Part print with two shaded views. Sizes in mm from the minimum x, y, z corner. A direction names the side the tool comes from. Give positions to 0.01 mm unless a question says otherwise; leave off trailing zeros. Order: outer loops, then holes, each group sorted by start corner. A loop starts at its lowest first (then second) coordinate and runs counter-clockwise, first axis right, second up. Notation, with made-up numbers: (54, -34.5) -> (76, -34.5) arc R31 cw to (76, 0.5) -> close; hole circle Ø6 at (-25, -40). An arc over 180 degrees is marked (long way). Answer as CSV lines item,"result".
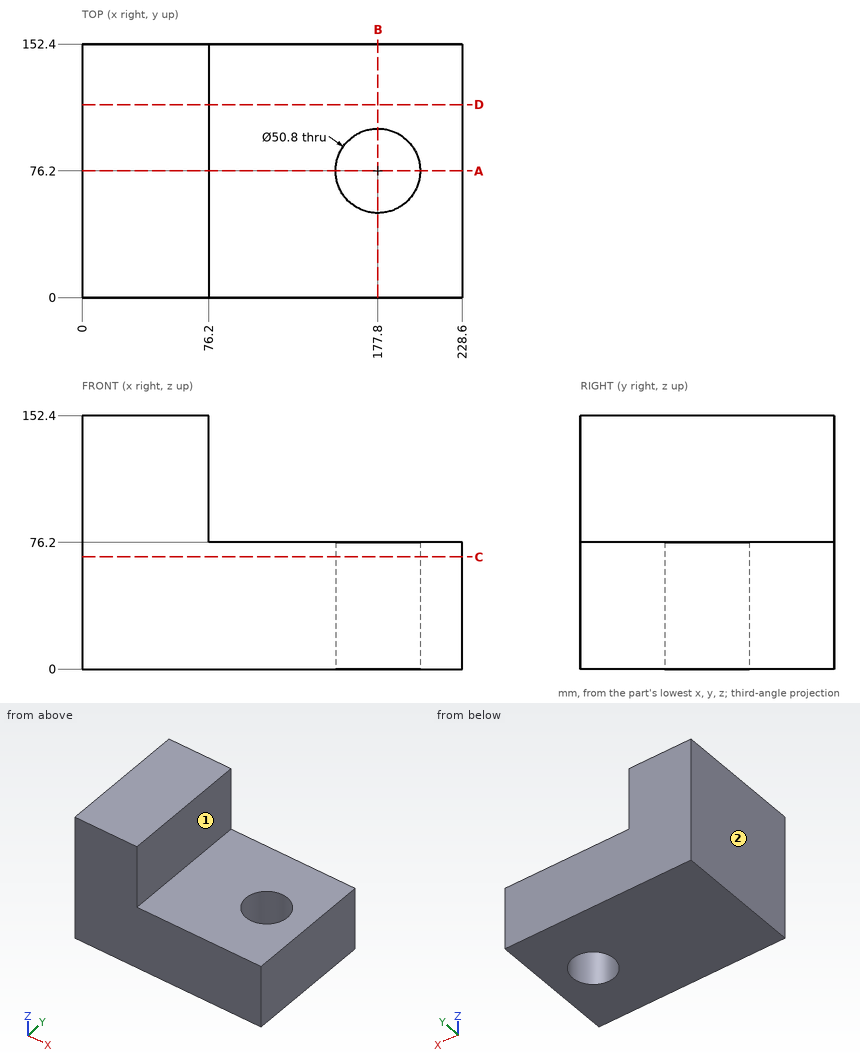
1) Which spindle directions (+Z, -Z, +X, -X, +Y, -Y) get a long thin tool onto all of the face, cutting with end or side? Do the marked faces 1 and 2. Say none if no direction does.
Data:
face 1,"+Z, +X, +Y, -Y"
face 2,"+Z, -Z, -X, +Y, -Y"
2) Wall check: line 1 along Y through (x, z) = (177.8, 44.5); line 2 along X through (y, z) = (40, 91.5); line 3 along X through (y, z) = (76, 48). Give the ranges that are in metal, low to high. Write a range as [from, to].
Data:
line 1,"y = [0, 50.8], [101.6, 152.4]"
line 2,"x = [0, 76.2]"
line 3,"x = [0, 152.4], [203.2, 228.6]"
3) Band-saw the part on A-A, the plane y = 76.2. Write the cut outline in (x, z), then the cut area to 3 significant figures.
Data:
outline,"(0, 0) -> (152.4, 0) -> (152.4, 76.2) -> (76.2, 76.2) -> (76.2, 152.4) -> (0, 152.4) -> close; (203.2, 0) -> (228.6, 0) -> (228.6, 76.2) -> (203.2, 76.2) -> close"
area,"19,400 mm2"
4) Band-saw the part on C-C, the plane z = 67.5. Write the cut outline in (x, y).
Data:
outline,"(0, 0) -> (228.6, 0) -> (228.6, 152.4) -> (0, 152.4) -> close; hole circle Ø50.8 at (177.8, 76.2)"
5) Band-saw the part on B-B, the plane x = 177.8. Write the cut outline in (y, z), then the cut area to 3 significant figures.
Data:
outline,"(0, 0) -> (50.8, 0) -> (50.8, 76.2) -> (0, 76.2) -> close; (101.6, 0) -> (152.4, 0) -> (152.4, 76.2) -> (101.6, 76.2) -> close"
area,"7,740 mm2"
6) Band-saw the part on D-D, the plane y = 116. Write the cut outline in (x, z).
Data:
outline,"(0, 0) -> (228.6, 0) -> (228.6, 76.2) -> (76.2, 76.2) -> (76.2, 152.4) -> (0, 152.4) -> close"
7) Pin check, flat tips, straight feed: P1, Ø10, axis at y = 39, z = 84.5, coming from the +X side; P2, Ø4, axis at x = 173.5, y = 38, coming from the +Z side. Stop position of each tip, or through.
Data:
P1,"stops at x = 76.2"
P2,"stops at z = 76.2"
